The drawing under review shows one solid part. Ordinate dimensions are in mm from its lowest x, y, z. A direction names the side the tool comes from. Coordinates: 2 decimals unless noted, no trailing zeros. Order: outer loops, then holes, each group sorted by start corner. A loop starts at its lowest first (then second) coordinate and runs counter-clockwise, first axis right, second up. Notation, with made-up numbers: (5.5, 62.25) -> (51.5, 62.25) arc R27 cw to (51.5, 93.25) -> close; hole circle Ø4 at (47, 87.5). An arc over 180 degrees is marked (long way). Use one line per item in the form item = value.
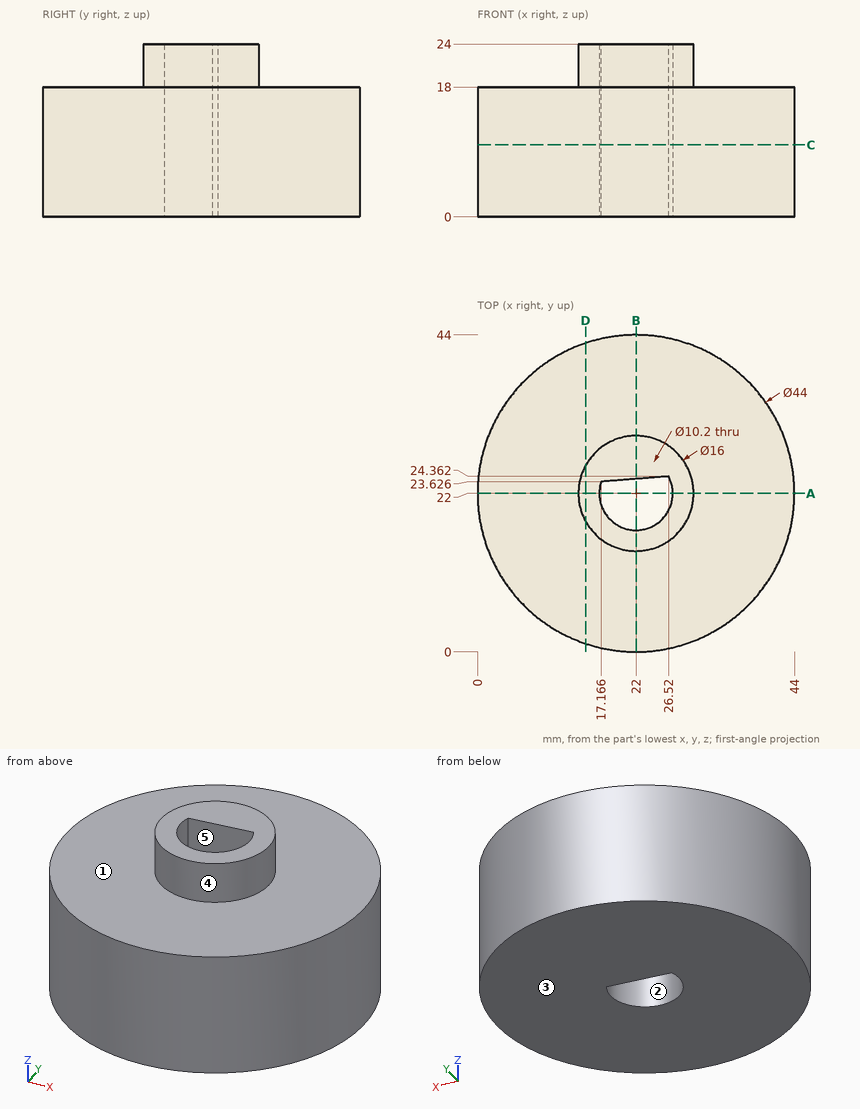
Item 1: Draft analysis for pull direction Y (two halves, no side actions). For the marked faces 3, 4 and 5, state which applies: released by +Y, released by -Y, zero draft, split by the parting line, or undercut.
Results found:
face_3 = zero draft
face_4 = split by the parting line
face_5 = undercut
Item 2: Clearance check with flat-ended pins moving along their axes: pin 1 (1.5 mm diameter, centred on x = 11, y = 18.5, fed in from +Z); pin 2 (4 mm diameter, centred on x = 26, z = 7.5, fed in from -Y); pin 3 (2 mm diameter, centred on x = 28, z = 5.5, fed in from +Y). State where each tip first meets the part, or that it passes through.
Results found:
pin_1 = 18
pin_2 = 0.09
pin_3 = 43.42
Item 3: We need section C-C (z = 10). Write out the cut boundary in (x, y).
Results found:
outline = circle Ø44 at (22, 22); hole (17.17, 23.63) arc R5.1 ccw (long way) to (26.52, 24.36) -> close
Item 4: We need section A-A (y = 22). Write out the cut boundary in (x, z), plus the area to 3 significant figures.
Results found:
outline = (0, 0) -> (16.9, 0) -> (16.9, 24) -> (14, 24) -> (14, 18) -> (0, 18) -> close; (27.1, 0) -> (44, 0) -> (44, 18) -> (30, 18) -> (30, 24) -> (27.1, 24) -> close
area = 643 mm²
Item 5: To check wall thickness, follow L1, parallel to Y at x = 22, z = 15.25; L2, parallel to Y at x = 22, z = 18.75; L3, parallel to Z at x = 18.5, y = 9. State the ranges of each line that lie inside material, in increasing order. Write a range as from..to.
Results found:
L1 = 0..16.9, 24.01..44
L2 = 14..16.9, 24.01..30
L3 = 0..18
Item 6: We need section B-B (x = 22). Write out the cut boundary in (y, z).
Results found:
outline = (0, 0) -> (16.9, 0) -> (16.9, 24) -> (14, 24) -> (14, 18) -> (0, 18) -> close; (24.01, 0) -> (44, 0) -> (44, 18) -> (30, 18) -> (30, 24) -> (24.01, 24) -> close
Item 7: Tool access review of the marked faces 1 and 2: name each direction out of +Z, -Z, +X, -X, +Y, -Y from which nothing blocks a thin tool from reaching the whole face with its end or side.
Results found:
face_1 = +Z
face_2 = +Z, -Z
Item 8: We need section D-D (x = 15). Write out the cut boundary in (y, z).
Results found:
outline = (1.14, 0) -> (42.86, 0) -> (42.86, 18) -> (25.87, 18) -> (25.87, 24) -> (18.13, 24) -> (18.13, 18) -> (1.14, 18) -> close
